The figure shows three views and two pictorial views of one solid part (mm, origin at its lowest corner). Answer the questions. A direction names the side the tool comes from. Give positions to 0.01 mm unless a question says otherwise; leave off trailing zeros. Loops run counter-clockwise (first coordinate to the right, second up) from the corner with the lowest first, then second, coordinate; pieces in that order, holes last. Notation, with made-up numbers: (45.5, 20.25) - (73.5, 20.25) arc R27 cw to (73.5, 41.25) - close; hole circle Ø2 at (85.5, 5.25). An arc over 180 degrees is marked (long way). One line per question, with ' | ' between items.
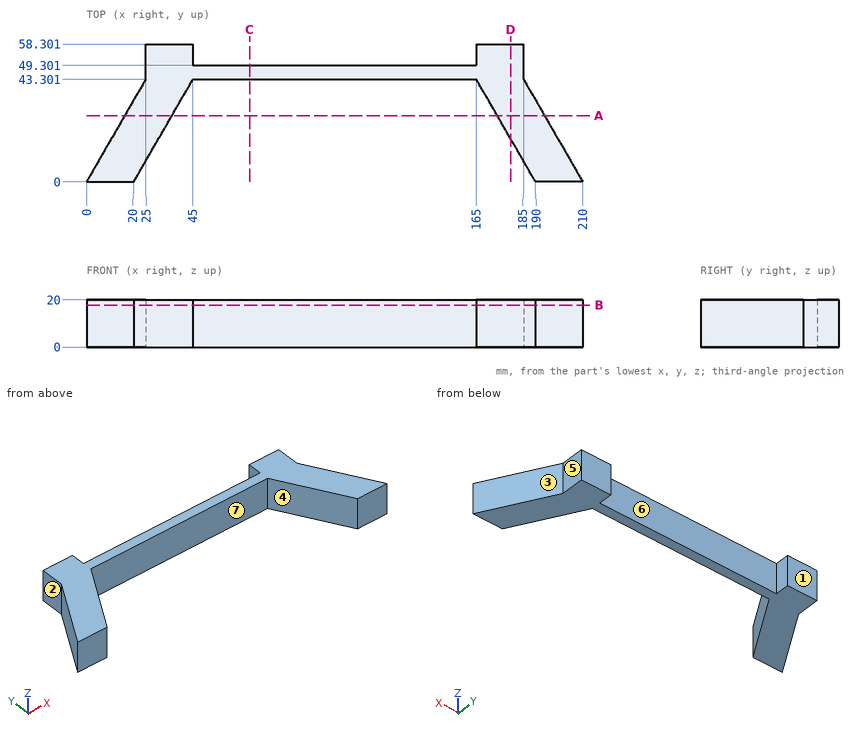
1. Which of the six approach directions +Z, -Z, +X, -X, +Y, -Y give full straight-line access (tool end or side, diameter ignored) to the marked faces 5, 6 and 7?
Evaluation:
face 5: +Z, -Z, +X, +Y | face 6: +Z, -Z, +Y | face 7: +Z, -Z, -Y
2. Consider L1, parallel to X at y = 50.5, z = 17.25; L2, parallel to X at y = 48, z = 13; L3, parallel to Y at x = 114.5, z = 15. Determine where each line is inside the solid, lowest interval first.
Evaluation:
L1: 25 to 45, 165 to 185 | L2: 25 to 185 | L3: 43.3 to 49.3
3. Find section A-A on y = 28. Write down the section's boundary in (x, z).
Evaluation:
outline: (16.17, 0) - (36.17, 0) - (36.17, 20) - (16.17, 20) - close; (173.83, 0) - (193.83, 0) - (193.83, 20) - (173.83, 20) - close
4. Find section D-D on x = 179.5. Write down the section's boundary in (y, z).
Evaluation:
outline: (18.19, 0) - (58.3, 0) - (58.3, 20) - (18.19, 20) - close
5. Find section C-C on x = 69. Write down the section's boundary in (y, z).
Evaluation:
outline: (43.3, 0) - (49.3, 0) - (49.3, 20) - (43.3, 20) - close
6. Flat-ended cylindrical pins translate along their axes: pin 1 (12 mm diameter, centred on y = 44.5, z = 3.5, fed in from -X); pin 2 (2 mm diameter, centred on x = 89.5, z = 17, fed in from -Y); pin 3 (4 mm diameter, centred on x = 155, z = 12, fed in from +Y). Find the tip coordinate at first contact, or state that the pin passes through.
Evaluation:
pin 1: x = 22.23 | pin 2: y = 43.3 | pin 3: y = 49.3
7. Find section B-B on z = 17.75. Write down the section's boundary in (x, y).
Evaluation:
outline: (0, 0) - (20, 0) - (45, 43.3) - (165, 43.3) - (190, 0) - (210, 0) - (185, 43.3) - (185, 58.3) - (165, 58.3) - (165, 49.3) - (45, 49.3) - (45, 58.3) - (25, 58.3) - (25, 43.3) - close
8. Determine the mould class of the marked faces 1, 2, 3 and 4 for opening direction X: +X half, -X half, draft (parallel to the pull), parting line (faces both ways), or undercut.
Evaluation:
face 1: draft | face 2: -X half | face 3: +X half | face 4: undercut
